Geometry: final body of the model. Coordinates: model frame, mm. Face numbers are marked on the shaded views. A direction names the side the tool comes from. Round coordinates to 2 decimals unless told otherwise and drop trailing zeros. Loops run counter-clockwise (first coordinate to the right, second up) from the corner with the lowest first, then second, coordinate; pieces in that order, holes last. Notation, with made-up numbers: M -8.5,-36.5 L 36.5,-36.5 A36 cw 36.5,-0.5 Z; hole C 25.5,29.25 d6. An arc over 180 degrees is marked long. Return JSON: item names as keys, results as strings.
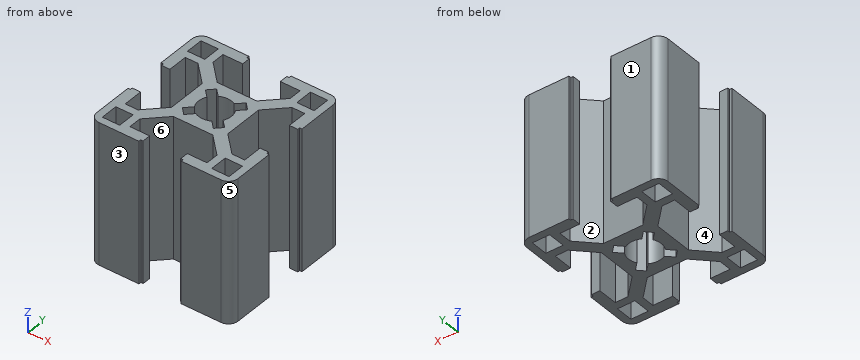
from build123d import *

# Parameters (mm, degrees)
SKETCH3_W           = 3.68
SKETCH3_H           = 3.68
BOSS_EXTRUDE1_DEPTH = 1219.2
SKETCH4_W           = 30
SKETCH4_H           = 2408.4
CUT_EXTRUDE1_DEPTH  = 1220.661280848


with BuildPart() as part:
    # Sketch3 → Boss-Extrude1 (new, symmetric)
    with BuildSketch(Plane.XY):
        with BuildLine():
            Line((-4.203948776, 6), (0, 6))
            Line((0, 6), (4.203948776, 6))
            Line((4.203948776, 6), (8.2, 9.996051224))
            Line((8.2, 9.996051224), (8.2, 12.71))
            Line((8.2, 12.71), (4, 12.71))
            Line((4, 12.71), (4, 14.5))
            Line((4, 14.5), (4.5, 14.5))
            Line((4.5, 14.5), (4.5, 15))
            Line((4.5, 15), (12.968, 15))
            ThreePointArc((12.968, 15), (14.404840979, 14.404840979), (15, 12.968))
            Line((15, 12.968), (15, 4.5))
            Line((15, 4.5), (14.5, 4.5))
            Line((14.5, 4.5), (14.5, 4))
            Line((14.5, 4), (12.71, 4))
            Line((12.71, 4), (12.71, 8.2))
            Line((12.71, 8.2), (9.996051224, 8.2))
            Line((9.996051224, 8.2), (6, 4.203948776))
            Line((6, 4.203948776), (6, 0))
            Line((6, 0), (6, -4.203948776))
            Line((6, -4.203948776), (9.996051224, -8.2))
            Line((9.996051224, -8.2), (12.71, -8.2))
            Line((12.71, -8.2), (12.71, -4))
            Line((12.71, -4), (14.5, -4))
            Line((14.5, -4), (14.5, -4.5))
            Line((14.5, -4.5), (15, -4.5))
            Line((15, -4.5), (15, -12.968))
            ThreePointArc((15, -12.968), (14.404840979, -14.404840979), (12.968, -15))
            Line((12.968, -15), (4.5, -15))
            Line((4.5, -15), (4.5, -14.5))
            Line((4.5, -14.5), (4, -14.5))
            Line((4, -14.5), (4, -12.71))
            Line((4, -12.71), (8.2, -12.71))
            Line((8.2, -12.71), (8.2, -9.996051224))
            Line((8.2, -9.996051224), (4.203948776, -6))
            Line((4.203948776, -6), (0, -6))
            Line((0, -6), (-4.203948776, -6))
            Line((-4.203948776, -6), (-8.2, -9.996051224))
            Line((-8.2, -9.996051224), (-8.2, -12.71))
            Line((-8.2, -12.71), (-4, -12.71))
            Line((-4, -12.71), (-4, -14.5))
            Line((-4, -14.5), (-4.5, -14.5))
            Line((-4.5, -14.5), (-4.5, -15))
            Line((-4.5, -15), (-12.968, -15))
            ThreePointArc((-12.968, -15), (-14.404840979, -14.404840979), (-15, -12.968))
            Line((-15, -12.968), (-15, -4.5))
            Line((-15, -4.5), (-14.5, -4.5))
            Line((-14.5, -4.5), (-14.5, -4))
            Line((-14.5, -4), (-12.71, -4))
            Line((-12.71, -4), (-12.71, -8.2))
            Line((-12.71, -8.2), (-9.996051224, -8.2))
            Line((-9.996051224, -8.2), (-6, -4.203948776))
            Line((-6, -4.203948776), (-6, 0))
            Line((-6, 0), (-6, 4.203948776))
            Line((-6, 4.203948776), (-9.996051224, 8.2))
            Line((-9.996051224, 8.2), (-12.71, 8.2))
            Line((-12.71, 8.2), (-12.71, 4))
            Line((-12.71, 4), (-14.5, 4))
            Line((-14.5, 4), (-14.5, 4.5))
            Line((-14.5, 4.5), (-15, 4.5))
            Line((-15, 4.5), (-15, 12.968))
            ThreePointArc((-15, 12.968), (-14.404840979, 14.404840979), (-12.968, 15))
            Line((-12.968, 15), (-4.5, 15))
            Line((-4.5, 15), (-4.5, 14.5))
            Line((-4.5, 14.5), (-4, 14.5))
            Line((-4, 14.5), (-4, 12.71))
            Line((-4, 12.71), (-8.2, 12.71))
            Line((-8.2, 12.71), (-8.2, 9.996051224))
            Line((-8.2, 9.996051224), (-4.203948776, 6))
        make_face()
        with Locations((-11.63, 11.63)):
            Rectangle(SKETCH3_W, SKETCH3_H, mode=Mode.SUBTRACT)
        with BuildLine():
            Line((-3.143089642, 4.493663594), (-1.705676589, 3.056250541))
            ThreePointArc((-1.705676589, 3.056250541), (0, 3.5), (1.705676589, 3.056250541))
            Line((1.705676589, 3.056250541), (3.143089642, 4.493663594))
            Line((3.143089642, 4.493663594), (4.493663594, 3.143089642))
            Line((4.493663594, 3.143089642), (3.056250541, 1.705676589))
            ThreePointArc((3.056250541, 1.705676589), (3.5, 0), (3.056250541, -1.705676589))
            Line((3.056250541, -1.705676589), (4.493663594, -3.143089642))
            Line((4.493663594, -3.143089642), (3.143089642, -4.493663594))
            Line((3.143089642, -4.493663594), (1.705676589, -3.056250541))
            ThreePointArc((1.705676589, -3.056250541), (0, -3.5), (-1.705676589, -3.056250541))
            Line((-1.705676589, -3.056250541), (-3.143089642, -4.493663594))
            Line((-3.143089642, -4.493663594), (-4.493663594, -3.143089642))
            Line((-4.493663594, -3.143089642), (-3.056250541, -1.705676589))
            ThreePointArc((-3.056250541, -1.705676589), (-3.5, 0), (-3.056250541, 1.705676589))
            Line((-3.056250541, 1.705676589), (-4.493663594, 3.143089642))
            Line((-4.493663594, 3.143089642), (-3.143089642, 4.493663594))
        make_face(mode=Mode.SUBTRACT)
        with Locations((11.63, 11.63)):
            Rectangle(SKETCH3_W, SKETCH3_H, mode=Mode.SUBTRACT)
        with Locations((11.63, -11.63)):
            Rectangle(SKETCH3_W, SKETCH3_H, mode=Mode.SUBTRACT)
        with Locations((-11.63, -11.63)):
            Rectangle(SKETCH3_W, SKETCH3_H, mode=Mode.SUBTRACT)
    extrude(amount=BOSS_EXTRUDE1_DEPTH, both=True)

    # Sketch4 → Cut-Extrude1 (cut, through all)
    with BuildSketch(Plane(origin=(0, 15, 0), x_dir=(1, 0, 0), z_dir=(0, 1, 0))):
        with Locations((0, 15)):
            Rectangle(SKETCH4_W, SKETCH4_H)
    extrude(amount=-CUT_EXTRUDE1_DEPTH, mode=Mode.SUBTRACT)


solid = part.part
Q1. Reachability of the marked faces 1 and 2 from +Z, -Z, +X, -X, +Y, -Y: full face, straight path, thin tool, end or side. Return the list, or none.
Determined:
{"face 1": "+Z, -Z, +X, -X, +Y", "face 2": "+Z, -Z"}
Q2. Section query D-D (z = 1202). State how many separate pieces and enclosed holes the cut face has, plus the area to 3 significant figures.
Determined:
{"separate pieces": "1", "enclosed holes": "5", "area": "337 mm^2"}
Q3. Section query B-B (x = -0.5). Output: boundary loops of the cut face in (y, z).
Determined:
{"outline": "M -6,1189.2 L -3.46,1189.2 L -3.46,1219.2 L -6,1219.2 Z; M 3.46,1189.2 L 6,1189.2 L 6,1219.2 L 3.46,1219.2 Z"}
Q4. Section query C-C (x = 6.5). Output: boundary loops of the cut face in (y, z), plus the area to 3 significant figures.
Determined:
{"outline": "M -15,1189.2 L -12.71,1189.2 L -12.71,1219.2 L -15,1219.2 Z; M -8.3,1189.2 L -4.7,1189.2 L -4.7,1219.2 L -8.3,1219.2 Z; M 4.7,1189.2 L 8.3,1189.2 L 8.3,1219.2 L 4.7,1219.2 Z; M 12.71,1189.2 L 15,1189.2 L 15,1219.2 L 12.71,1219.2 Z", "area": "353 mm^2"}
Q5. Pull-direction query (X, two-part tool) for the marked faces 3, 4, 5 and 6; classes: pulls with the +X half, pulls with the -X half, needs draft (parallel to the pull), parting line crosses it, or undercut.
Determined:
{"face 3": "needs draft", "face 4": "undercut", "face 5": "pulls with the +X half", "face 6": "undercut"}
Q6. Material intervals for L1, parallel to Y at x = 11, z = 1216; L2, parallel to X at y = 13, z = 1213.5, sorted ascending.
Determined:
{"L1": "y = -15 to -13.47, -9.79 to -8.2, 8.2 to 9.79, 13.47 to 15", "L2": "x = -15 to -13.47, -9.79 to -4, 4 to 9.79, 13.47 to 15"}
Q7. Pin query (flat end, axial travel): pin 1 (4 mm diameter, centred on y = 0.5, z = 1198, fed in from +X); pin 2 (0.6 mm diameter, centred on y = -4, z = 1200, fed in from +X). Return the tip coordinate at first contact, or that it passes through.
Determined:
{"pin 1": "stops at x = 6", "pin 2": "stops at x = 14.5"}
Q8. Section query A-A (y = -11.75). Output: boundary loops of the cut face in (x, z).
Determined:
{"outline": "M -15,1189.2 L -13.47,1189.2 L -13.47,1219.2 L -15,1219.2 Z; M -9.79,1189.2 L -8.2,1189.2 L -8.2,1219.2 L -9.79,1219.2 Z; M 8.2,1189.2 L 9.79,1189.2 L 9.79,1219.2 L 8.2,1219.2 Z; M 13.47,1189.2 L 15,1189.2 L 15,1219.2 L 13.47,1219.2 Z"}
